Study the drawing (mm; zero at the part's minimum x, y, z) and answer. Round coordinates to 2 decimals unless told otherwise and drop trailing zeros. Write each loop counter-clockwise with the first axis right and the second up, starting at its lowest first coordinate (ties: lowest second). Pieces come first, ordered by that corner, then holes. Notation, with made-up numbers: (76.25, 48.5) - (132.25, 48.5) arc R25 cw to (132.25, 73.5) - close; hole circle Ø7 at (45, 67). An arc over 180 degrees is marked (long way). Return JSON: item names as keys, results as strings. Group by question number.
(1) Section A-A, the plane x = 114.3 is taken. Write down the section's boundary in (y, z).
(2) Find the intervals of material crossed by line 1 along X through (y, z) = (3.25, 12.7); line 2 along Z through (x, y) = (114.3, 9.5); line 3 along X through (y, z) = (6, 13.5), in increasing order. Write a range as [from, to].
(3) This flat-tipped pin is pushed along its axis until it touches: pin 1 (3 mm diameter, centred on x = 69, y = 9, fed in from -Z). Where does it stop, or does it pass through?
(4) Section B-B, the plane z = 12.7 is taken. Write down the section's boundary in (x, y).
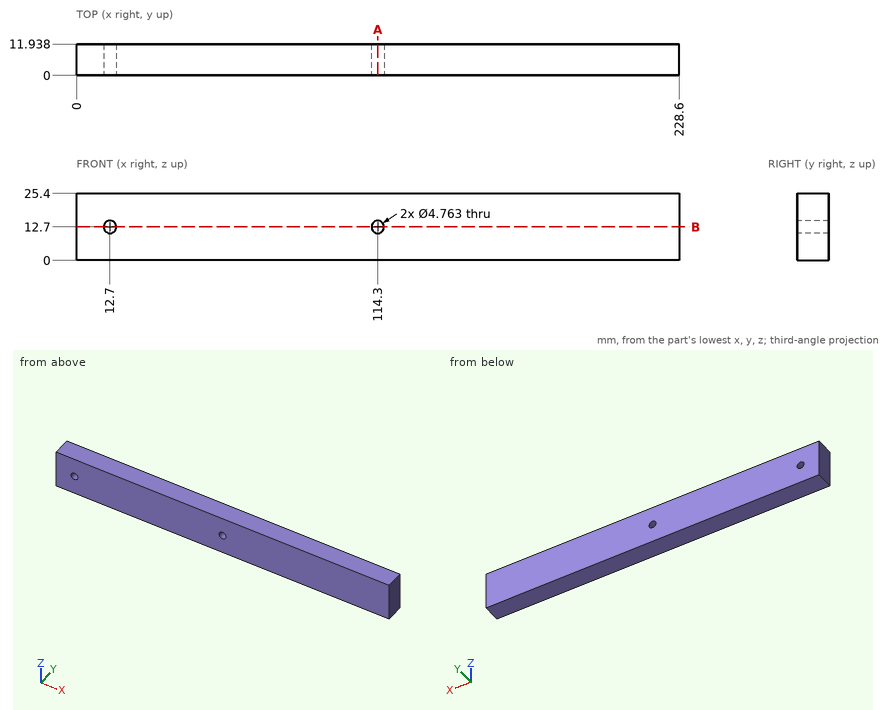
Working result:
{
 "1": {"outline": "(0, 0) - (11.94, 0) - (11.94, 10.32) - (0, 10.32) - close; (0, 15.08) - (11.94, 15.08) - (11.94, 25.4) - (0, 25.4) - close"},
 "2": {"line 1": "x = [0, 10.32], [15.08, 111.92], [116.68, 228.6]", "line 2": "z = [0, 10.32], [15.08, 25.4]", "line 3": "x = [0, 10.46], [14.94, 112.06], [116.54, 228.6]"},
 "3": {"pin 1": "stops at z = 0"},
 "4": {"outline": "(0, 0) - (10.32, 0) - (10.32, 11.94) - (0, 11.94) - close; (15.08, 0) - (111.92, 0) - (111.92, 11.94) - (15.08, 11.94) - close; (116.68, 0) - (228.6, 0) - (228.6, 11.94) - (116.68, 11.94) - close"}
}
